Check sheet for the modelled part. Datum: model origin and axes. Units: mm. A direction names the side the tool comes from. Round coordinates to 2 decimals unless told otherwise and drop trailing zeros. Write each loop counter-clockwise with the first axis right and the second up, starting at its lowest first coordinate (ties: lowest second). Pieces come first, ordered by that corner, then holes. Notation, with made-up numbers: (-1, 50) -> (30, 50) arc R20 ccw to (30, 77) -> close; hole circle Ø2 at (31, 24). An arc over 180 degrees is marked (long way). One line per item, written item: value.
from build123d import *

# Parameters (mm, degrees)
SKETCH_1_R      = 1.5
SKETCH_1_R_2    = 3.2
EXTRUDE_1_DEPTH = 2


with BuildPart() as part:
    # 草图1 → 凸台-拉伸1 (new body)
    with BuildSketch(Plane(origin=(0, 0, 0), x_dir=(1, 0, 0), z_dir=(0, 1, 0))):
        with BuildLine():
            ThreePointArc((-16.5, 3), (-19.5, 0), (-16.5, -3))
            Line((-16.5, -3), (-13.674794331, -3))
            ThreePointArc((-13.674794331, -3), (-7, -12.124355653), (4.239320954, -13.342719282))
            Line((4.239320954, -13.342719282), (5.651923789, -15.789419162))
            ThreePointArc((5.651923789, -15.789419162), (9.75, -16.887495374), (10.848076211, -12.789419162))
            Line((10.848076211, -12.789419162), (9.435473377, -10.342719282))
            ThreePointArc((9.435473377, -10.342719282), (14, 0), (9.435473377, 10.342719282))
            Line((9.435473377, 10.342719282), (10.848076211, 12.789419162))
            ThreePointArc((10.848076211, 12.789419162), (9.75, 16.887495374), (5.651923789, 15.789419162))
            Line((5.651923789, 15.789419162), (4.239320954, 13.342719282))
            ThreePointArc((4.239320954, 13.342719282), (-7, 12.124355653), (-13.674794331, 3))
            Line((-13.674794331, 3), (-16.5, 3))
        make_face()
        with Locations(Location((-16.5, 0, 0), (0, 0, 270))):
            Circle(SKETCH_1_R, mode=Mode.SUBTRACT)
        with Locations(Location((8.25, -14.289419162, 0), (0, 0, 270))):
            Circle(SKETCH_1_R, mode=Mode.SUBTRACT)
        with Locations(Location((0, 0, 0), (0, 0, 270))):
            Circle(SKETCH_1_R_2, mode=Mode.SUBTRACT)
        with Locations(Location((8.25, 14.289419162, 0), (0, 0, 270))):
            Circle(SKETCH_1_R, mode=Mode.SUBTRACT)
    extrude(amount=EXTRUDE_1_DEPTH)


solid = part.part
Item 1: Sectioned sample at B-B on y = 0.95. Enter the section's corners in (x, z).
Answer:
outline: (-16.5, -3) -> (-13.67, -3) arc R14 ccw to (4.24, -13.34) -> (5.65, -15.79) arc R3 ccw to (10.85, -12.79) -> (9.44, -10.34) arc R14 ccw to (9.44, 10.34) -> (10.85, 12.79) arc R3 ccw to (5.65, 15.79) -> (4.24, 13.34) arc R14 ccw to (-13.67, 3) -> (-16.5, 3) arc R3 ccw to start; hole circle Ø3 at (-16.5, 0); hole circle Ø6.4 at (0, 0); hole circle Ø3 at (8.25, -14.29); hole circle Ø3 at (8.25, 14.29)
Item 2: Tool access check on faces 5 (the flat face through (-15, 1, 3)), 6 (the flat face through (10.132, 0.986, -11.549)), 7 (the flat face through (4.956, 0.986, -14.583)), 8 (the cylindrical face through (9.81, 0.99, -16.85)). Record the directions out of +Z, -Z, +X, -X, +Y, -Y that give a thin tool (end or side, any length) a straight path to the whole face; none if there is none.
Answer:
face 5: +Z, -X, +Y, -Y
face 6: +X, +Y, -Y
face 7: -Z, +Y, -Y
face 8: +Y, -Y
Item 3: Thickness scan on line 1 (X direction, y = 1.15, z = 0); line 2 (Z direction, x = 11, y = 0.8); line 3 (X direction, y = 1.45, z = -1). Record the ranges inside material, lowest first.
Answer:
line 1: x = -19.5 to -18, -15 to -3.2, 3.2 to 14
line 2: z = -15.49 to -13.09, -8.66 to 8.66, 13.09 to 15.49
line 3: x = -19.33 to -17.62, -15.38 to -3.04, 3.04 to 13.96
Item 4: Depth check by flat-ended pin: P1, Ø1, axis at x = -14.5, z = -5, coming from the -Y side; P2, Ø0.6, axis at x = -15, y = 1.5, coming from the -Z side; P3, Ø1, axis at y = 1.5, z = -2.5, coming from the -X side. Enter the tip coordinate at first touch or a pass-through.
Answer:
P1: passes through
P2: stops at z = -3
P3: stops at x = -18.74
Item 5: Sectioned sample at A-A on x = 8.25. Enter the section's corners in (y, z).
Answer:
outline: (0, -17.29) -> (2, -17.29) -> (2, -15.79) -> (0, -15.79) -> close; (0, -12.79) -> (2, -12.79) -> (2, 12.79) -> (0, 12.79) -> close; (0, 15.79) -> (2, 15.79) -> (2, 17.29) -> (0, 17.29) -> close
Item 6: Sectioned sample at D-D on x = 0. Enter the section's corners in (y, z), and give its area (3 significant figures).
Answer:
outline: (0, -14) -> (2, -14) -> (2, -3.2) -> (0, -3.2) -> close; (0, 3.2) -> (2, 3.2) -> (2, 14) -> (0, 14) -> close
area: 43.2 mm^2
Item 7: Sectioned sample at C-C on z = 0. Enter the section's corners in (x, y), and give its area (3 significant figures).
Answer:
outline: (-19.5, 0) -> (-18, 0) -> (-18, 2) -> (-19.5, 2) -> close; (-15, 0) -> (-3.2, 0) -> (-3.2, 2) -> (-15, 2) -> close; (3.2, 0) -> (14, 0) -> (14, 2) -> (3.2, 2) -> close
area: 48.2 mm^2
Item 8: Mould release check, pull along Z, two halves, no side actions. Record for faces 1 (the cylindrical face through (7.68, 0.99, -12.9)), 2 (the flat face through (-15, 1, -3)), 3 (the flat face through (4.936, 0.986, 14.549)), 4 (the cylindrical face through (-19.5, 1, -0.1)): pulls with the +Z half, pulls with the -Z half, needs draft (parallel to the pull), parting line crosses it, or undercut.
Answer:
face 1: undercut
face 2: pulls with the -Z half
face 3: pulls with the +Z half
face 4: parting line crosses it
